Input: part model. Units: mm. Frame: model coordinates. A direction names the side the tool comes from. Give positions to 0.01 mm unless a question says otherwise; leave off trailing zeros. Loops run counter-clockwise (first coordinate to the right, second up) from the corner with the lowest first, then second, coordinate; pieces in that order, holes last. Notation, with made-up numbers: M 83,-5 L 118,-5 A37 ccw 118,34 Z; hole C 54.25,86 d1. An arc over 180 degrees is marked long. Return JSON: item names as keys, results as strings. Group by question number.
Autodesk Inventor part; units mm, degrees
ref_plane "YZ Plane" through (0, 0, 0) normal (1, 0, 0) x (0, 1, 0)
ref_plane "XZ Plane" through (0, 0, 0) normal (0, 1, 0) x (-1, 0, 0)
ref_plane "XY Plane" through (0, 0, 0) normal (0, 0, 1) x (1, 0, 0)
sketch "Sketch1" plane through (0, 0, 0) normal (0, 0, 1) x (1, 0, 0)
  line L0 (0, 0) -> (4, 0)
  line L1 (4, 0) -> (4, 4)
  line L2 (4, 4) -> (0, 4)
  line L3 (0, 4) -> (0, 0)
  line L4 (-0.4, -1.4) -> (4.4, -1.4)
  line L5 (5.4, -0.4) -> (5.4, 5.4)
  line L6 (5.4, 5.4) -> (-0.4, 5.4)
  line L7 (-1.4, 4.4) -> (-1.4, -0.4)
  arc A0 (-0.4, 5.4) -> (-1.4, 4.4) centre (-0.4, 4.4) ccw
  arc A1 (-1.4, -0.4) -> (-0.4, -1.4) centre (-0.4, -0.4) ccw
  arc A2 (4.4, -1.4) -> (5.4, -0.4) centre (4.4, -0.4) ccw
  point P0 (-1.4, -1.4)
  point P1 (5.4, -1.4)
  point P2 (-1.4, 5.4)
  dimension "d0" = 4
  dimension "d1" = 4
  dimension "d2" = 1.4
  dimension "d5" = 1
extrude "Extrusion1" add sketch "Sketch1" along normal blind 2.5
sketch "草圖3" plane through (4, 4, 0) normal (-1, 0, 0) x (0, 0, 1)
  line L0 (2.5, 0) -> (2.5, -4)
  line L1 (-0.5, 2.3) -> (3, 2.3)
  line L2 (3.5, 1.8) -> (3.5, -0.4)
  line L3 (3, -0.9) -> (-0.5, -0.9)
  line L4 (-1, -0.4) -> (-1, 1.8)
  line L5 (0, -5.4) -> (2.5, -5.4)
  arc A0 (-0.5, 2.3) -> (-1, 1.8) centre (-0.5, 1.8) ccw
  arc A1 (-1, -0.4) -> (-0.5, -0.9) centre (-0.5, -0.4) ccw
  arc A2 (3, -0.9) -> (3.5, -0.4) centre (3, -0.4) ccw
  arc A3 (3.5, 1.8) -> (3, 2.3) centre (3, 1.8) ccw
  point P0 (-1, 2.3)
  point P1 (3.5, -0.9)
  point P2 (3.5, 2.3)
  dimension "d14" = 4.5
  dimension "d16" = 3.2
  dimension "d17" = 4.5
  dimension "d18" = 1
  dimension "d19" = 0.5
extrude "擠出3" add sketch "草圖3" against normal blind 3 draft -5
properties part number "fastener_04"
Item 1: Reachability of faces 5 (the face through (5.4, 1, 1)), 6 (the face through (0, 2, 1)), 7 (the face through (2, 5.4, 1)), 8 (the face through (2, -1.4, 1)) from +Z, -Z, +X, -X, +Y, -Y: full face, straight path, thin tool, end or side. Return the list, or none.
Item 2: Pull-direction query (X, two-part tool) for faces 1 (the face through (2, 0, 1)), 2 (the face through (-0.3, 2, 2.5)), 3 (the face through (4, 3, 1)), 4 (the face through (5.81, 3.26, 1.27)); classes: pulls with the +X half, pulls with the -X half, needs draft (parallel to the pull), parting line crosses it, or undercut.
Item 3: Section B-B, the plane z = 0.4. Return loops of the section in (x, y).
Item 4: Section A-A, the plane y = 2.75. Return loops of the section in (x, z), then the cut area to 3 significant figures.
Item 5: First-contact query: pin 1 Ø1.5 at (x, y) = (3, 0) entering from -Z; pin 2 Ø2 at (x, y) = (1, 4.5) entering from +Z; pin 3 Ø2 at (y, z) = (2, 1) entering from +X. Flat tips, straight axial feed; report the tip coordinate or a pass-through.
Item 6: Section D-D, the plane x = 5.75. Return loops of the section in (y, z), then the cut area to 3 significant figures.
Item 7: Material intervals for line 1 (X direction, y = 0.25, z = 2.3); line 2 (X direction, y = 3.5, z = -0.55), sorted ascending. Write a range as from..to.
Answer below:
{
 "1": {"face 5": "+Z, -Z, +X, -Y", "face 6": "+Z, -Z", "face 7": "+Z, -Z, -X, +Y", "face 8": "+Z, -Z, +X, -X, -Y"},
 "2": {"face 1": "undercut", "face 2": "needs draft", "face 3": "undercut", "face 4": "pulls with the +X half"},
 "3": {"outline": "M -1.4,-0.4 A1 ccw -0.4,-1.4 L 4.4,-1.4 A1 ccw 5.4,-0.4 L 5.4,3.22 L 7,3.36 L 7,6.04 L 4,6.3 L 4,5.4 L -0.4,5.4 A1 ccw -1.4,4.4 Z; hole M 0,0 L 4,0 L 4,4 L 0,4 Z"},
 "4": {"outline": "M -1.4,0 L 0,0 L 0,2.5 L -1.4,2.5 Z; M 4,0 L 5.4,0 L 5.4,2.5 L 4,2.5 Z", "area": "7.00 mm^2"},
 "5": {"pin 1": "z = 0", "pin 2": "z = 2.5", "pin 3": "x = 5.4"},
 "6": {"outline": "M 3.25,-0.5 A0.35 ccw 3.6,-0.85 L 5.8,-0.85 A0.35 ccw 6.15,-0.5 L 6.15,3 A0.35 ccw 5.8,3.35 L 3.6,3.35 A0.35 ccw 3.25,3 Z", "area": "12.0 mm^2"},
 "7": {"line 1": "-1.4..0, 4..5.4", "line 2": "4..7"}
}
